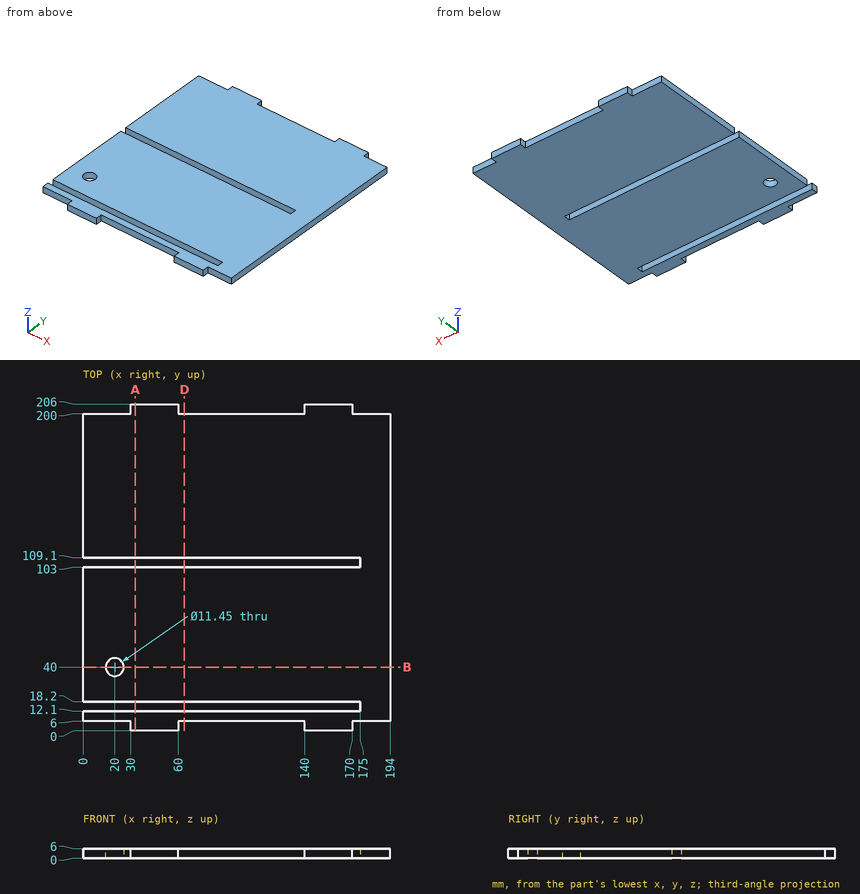
Design review of the part shown in the three views and the two pictorial views. Dimensions are in mm from the part's minimum x, y and z. Round coordinates to 2 decimals unless told otherwise and drop trailing zeros. Loops run counter-clockwise (first coordinate to the right, second up) from the corner with the lowest first, then second, coordinate; pieces in that order, holes last. Notation, with made-up numbers: M 20,22.25 L 63,22.25 A22 ccw 63,36.25 Z; hole C 75,51 d8. An arc over 180 degrees is marked long. Write item = value, one per line.
Item 1: Insertion check: P1, Ø3, axis at x = 22, z = 4, coming from the +Y side; P2, Ø3, axis at y = 15, z = 3, coming from the -X side; P3, Ø3, axis at x = 22, z = 3.5, coming from the -Y side. Each pin has a flat end and moves straight along its axis. Give the tip position at first contact, or say it passes through.
Return value:
P1 = 200
P2 = 175
P3 = 6
Item 2: Take a section at A-A on x = 33. Write out the cut boundary in (y, z), then the cut area to 3 significant figures.
Return value:
outline = M 0,0 L 12.1,0 L 12.1,6 L 0,6 Z; M 18.2,0 L 103,0 L 103,6 L 18.2,6 Z; M 109.1,0 L 206,0 L 206,6 L 109.1,6 Z
area = 1,160 mm2
Item 3: Take a section at B-B on y = 40. Write out the cut boundary in (x, z) (3 decimals), then the cut area to 3 significant figures.
Return value:
outline = M 0,0 L 14.275,0 L 14.275,6 L 0,6 Z; M 25.725,0 L 194,0 L 194,6 L 25.725,6 Z
area = 1,100 mm2
Item 4: Take a section at D-D on x = 64. Write out the cut boundary in (y, z), then the cut area to 3 significant figures.
Return value:
outline = M 6,0 L 12.1,0 L 12.1,6 L 6,6 Z; M 18.2,0 L 103,0 L 103,6 L 18.2,6 Z; M 109.1,0 L 200,0 L 200,6 L 109.1,6 Z
area = 1,090 mm2
Item 5: For line 1 (Y direction, x = 77, z = 5.7); line 2 (Y direction, x = 37.5, z = 5.7); line 3 (Y direction, x = 20, z = 2.9) (3 decimals), list the stretches that pass through material, from the lowest coordinate up. Write a range as [from, to].
Return value:
line_1 = [6, 12.1], [18.2, 103], [109.1, 200]
line_2 = [0, 12.1], [18.2, 103], [109.1, 206]
line_3 = [6, 12.1], [18.2, 34.275], [45.725, 103], [109.1, 200]
